Design review of the part built by this model. Coordinates are the model's own, in mm. Coordinates: 2 decimals unless noted, no trailing zeros. Order: outer loops, then holes, each group sorted by start corner. A loop starts at its lowest first (then second) coordinate and runs counter-clockwise, first axis right, second up. Notation, with made-up numbers: M 28.25,-20 L 59.25,-20 A11 cw 59.25,-8 Z; hole C -30,-15.5 d1. An arc over 180 degrees is marked long. Answer in a Markdown table with one row per item.
from build123d import *

# Parameters (mm, degrees)
ESQUISSE1_R             = 12.5
BOSS_EXTRU_1_DEPTH      = 326
ESQUISSE2_R             = 15
BOSS_EXTRU_2_DEPTH      = 16
BOSS_EXTRU_4_START      = -310
ESQUISSE2_2_R           = 15
BOSS_EXTRU_4_DEPTH      = 16
ESQUISSE3_R             = 11
BOSS_EXTRU_5_DEPTH      = 21
ESQUISSE4_W             = 5
ESQUISSE4_H             = 22
ENL_V_MAT_EXTRU_1_DEPTH = 19
ESQUISSE5_R             = 4
ENL_V_MAT_EXTRU_2_DEPTH = 328.1543978
BOSS_EXTRU_6_START      = 14
ESQUISSE6_R             = 11
BOSS_EXTRU_6_DEPTH      = 14
CHANFREIN1_SIZE         = 1
ESQUISSE7_R             = 5.25
ENL_V_MAT_EXTRU_3_DEPTH = 250


with BuildPart() as part:
    # Esquisse1 → Boss.-Extru.1 (new body)
    with BuildSketch(Plane.XY):
        Circle(ESQUISSE1_R)
    extrude(amount=BOSS_EXTRU_1_DEPTH)

    # Esquisse2 → Boss.-Extru.2 (add)
    with BuildSketch(Plane.XY.offset(326)):
        Circle(ESQUISSE2_R)
    extrude(amount=-BOSS_EXTRU_2_DEPTH)

    # Esquisse2_2 → Boss.-Extru.4 (add)
    with BuildSketch(Plane.XY.offset(326).offset(BOSS_EXTRU_4_START)):
        Circle(ESQUISSE2_2_R)
    extrude(amount=-BOSS_EXTRU_4_DEPTH)

    # Esquisse3 → Boss.-Extru.5 (add)
    with BuildSketch(Plane(origin=(0, 0, 0), x_dir=(-1, 0, 0), z_dir=(0, 0, -1))):
        with Locations(Location((0, 0, 0), (0, 0, 180))):
            Circle(ESQUISSE3_R)
    extrude(amount=BOSS_EXTRU_5_DEPTH)

    # Esquisse4 → Enl_v. mat.-Extru.1 (cut)
    with BuildSketch(Plane(origin=(0, 0, -21), x_dir=(-1, 0, 0), z_dir=(0, 0, -1))):
        with Locations((-10.5, 0)):
            Rectangle(ESQUISSE4_W, ESQUISSE4_H)
        with Locations((10.5, 0)):
            Rectangle(ESQUISSE4_W, ESQUISSE4_H)
    extrude(amount=-ENL_V_MAT_EXTRU_1_DEPTH, mode=Mode.SUBTRACT)

    # Esquisse5 → Enl_v. mat.-Extru.2 (cut, through all)
    with BuildSketch(Plane(origin=(8, 0, 0), x_dir=(0, 0, -1), z_dir=(1, 0, 0))):
        with Locations((12, 0)):
            Circle(ESQUISSE5_R)
    extrude(amount=-ENL_V_MAT_EXTRU_2_DEPTH, mode=Mode.SUBTRACT)

    # Esquisse6 → Boss.-Extru.6 (add)
    with BuildSketch(Plane.XY.offset(326).offset(BOSS_EXTRU_6_START)):
        Circle(ESQUISSE6_R)
    extrude(amount=-BOSS_EXTRU_6_DEPTH)

    # Chanfrein1
    chanfrein1_edges = [part.edges().sort_by_distance(p)[0] for p in [
        (0, -11, -21),
        (8, 0, -2),
        (0, 11, -21),
        (-8, 0, -2),
        (-11, 0, 340),
    ]]
    chamfer(chanfrein1_edges, length=CHANFREIN1_SIZE)

    # Esquisse7 → Enl_v. mat.-Extru.3 (cut)
    with BuildSketch(Plane.XY.offset(340)):
        Circle(ESQUISSE7_R)
    extrude(amount=-ENL_V_MAT_EXTRU_3_DEPTH, mode=Mode.SUBTRACT)


solid = part.part
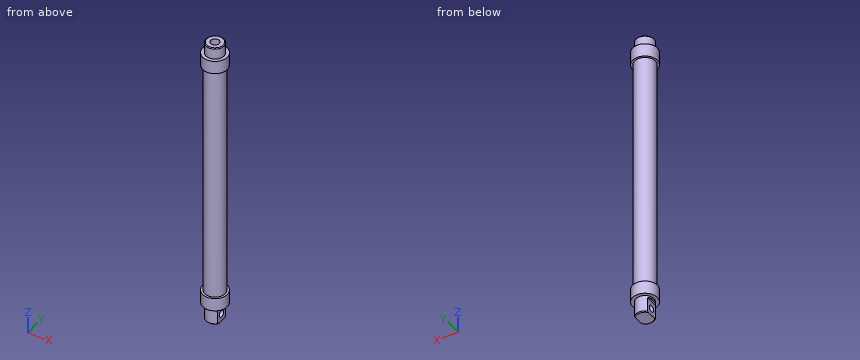
(1) Insertion check: pin 1 Ø3 at (y, z) = (8.5, 52.5) entering from -X; pin 2 Ø5 at (y, z) = (0, -12) entering from -X; pin 3 Ø5 at (y, z) = (-4, 143) entering from +X; pin 4 Ø5 at (x, z) = (2.5, 44) entering from -Y. Each pin has a flat end and moves straight along its axis. Give the tip position at first contact, or say it passes through.
Return value:
| item | result |
|---|---|
| pin 1 | stops at x = -10.36 |
| pin 2 | passes through |
| pin 3 | stops at x = 12.41 |
| pin 4 | stops at y = -12.5 |
(2) Add section A-A, the plane z = -12. Give the boundary of the cut face in (x, y), and give its area (3 significant figures).
Return value:
| item | result |
|---|---|
| outline | M -8,-7.55 A11 ccw 8,-7.55 L 8,-4 L -8,-4 Z; M -8,4 L 8,4 L 8,7.55 A11 ccw -8,7.55 Z |
| area | 190 mm2 |
(3) Add section C-C, the plane z = 259.5. Give the boundary of the cut face in (x, y), and give its area (3 significant figures).
Return value:
| item | result |
|---|---|
| outline | C 0,0 d25; hole C 0,0 d10.5 |
| area | 404 mm2 |
(4) For line 1 along Z through (x, y) = (-11.5, 9.5); line 2 along Y through (x, z) = (0, 184); line 3 along X through (y, z) = (0.25, 281), list the stretches that pass through material, from the lowest coordinate up. Write a range as from..to.
Return value:
| item | result |
|---|---|
| line 1 | z = 0..16, 310..326 |
| line 2 | y = -12.5..-5.25, 5.25..12.5 |
| line 3 | x = -12.5..-5.24, 5.24..12.5 |
